Could you check a few things on this model? Use its own coordinates, in mm. A direction names the side the tool comes from. Round coordinates to 2 decimals unless told otherwise and drop trailing zeros. Loops run counter-clockwise (first coordinate to the right, second up) from the corner with the lowest first, then second, coordinate; pieces in that order, holes last. Notation, with made-up numbers: M 64,83 L 111,83 A28 cw 111,114 Z; hole C 2,55 d1. An arc over 180 degrees is marked long. Answer in a Markdown table with one row per item.
```python
from build123d import *

# Parameters (mm, degrees)
SKETCH_1_W          = 40
SKETCH_1_H          = 32
SKETCH_1_R          = 14
SKETCH_1_R_2        = 1.6
EXTRUDE_1_DEPTH     = 24
SKETCH_3_W          = 30.4
SKETCH_3_H          = 51.000805287
CUT_EXTRUDE_2_DEPTH = 22.4
SKETCH_4_W          = 6.12991639
SKETCH_4_H          = 19.114193836
CUT_EXTRUDE_3_DEPTH = 57.568542495
FILLET_1_R          = 1
SKETCH_6_W          = 15.6
SKETCH_6_H          = 32
EXTRUDE_3_DEPTH     = 10
SKETCH_8_R          = 1.6
CUT_EXTRUDE_4_DEPTH = 66.604877867
CUT_EXTRUDE_5_DEPTH = 66.604877867
CHAMFER_1_SIZE      = 1
SKETCH_10_W         = 3.521220791
SKETCH_10_H         = 7.290414878
CUT_EXTRUDE_6_DEPTH = 15
SKETCH_11_W         = 3.883261803
SKETCH_11_H         = 7.637577492
CUT_EXTRUDE_7_DEPTH = 11


with BuildPart() as part:
    # 草图1 → 凸台-拉伸1 (new body)
    with BuildSketch(Plane.XY):
        with Locations((-20, 16)):
            Rectangle(SKETCH_1_W, SKETCH_1_H)
        with Locations((-20, 16)):
            Circle(SKETCH_1_R, mode=Mode.SUBTRACT)
        with Locations((-2.64, 14.11)):
            Circle(SKETCH_1_R_2, mode=Mode.SUBTRACT)
        with Locations(Location((-37.36, 14.11, 0), (0, 0, 180))):
            Circle(SKETCH_1_R_2, mode=Mode.SUBTRACT)
    extrude(amount=EXTRUDE_1_DEPTH)

    # 草图3 → 切除-拉伸2 (cut)
    with BuildSketch(Plane(origin=(0, 0, 0), x_dir=(-1, 0, 0), z_dir=(0, 0, -1))):
        with Locations((20, 12.05288799)):
            Rectangle(SKETCH_3_W, SKETCH_3_H)
    extrude(amount=-CUT_EXTRUDE_2_DEPTH, mode=Mode.SUBTRACT)

    # 草图4 → 切除-拉伸3 (cut, through all)
    with BuildSketch(Plane(origin=(0, 0, 0), x_dir=(-1, 0, 0), z_dir=(0, 0, -1))):
        with Locations((0.535041805, 26.667096918)):
            Rectangle(SKETCH_4_W, SKETCH_4_H)
        with Locations((39.464958195, 26.667096918)):
            Rectangle(SKETCH_4_W, SKETCH_4_H)
        with Locations((39.464958195, 1.552903082)):
            Rectangle(SKETCH_4_W, SKETCH_4_H)
        with Locations((0.535041805, 1.552903082)):
            Rectangle(SKETCH_4_W, SKETCH_4_H)
    extrude(amount=-CUT_EXTRUDE_3_DEPTH, mode=Mode.SUBTRACT)

    # 圆角1
    fillet_1_edges = [part.edges().sort_by_distance(p)[0] for p in [
        (0, 11.11, 12),
        (0, 17.11, 12),
        (-40, 17.11, 12),
        (-40, 11.11, 12),
    ]]
    fillet(fillet_1_edges, radius=FILLET_1_R)

    # 草图6 → 凸台-拉伸3 (add)
    with BuildSketch(Plane.XY.offset(24)):
        with Locations((-44.2, 16)):
            Rectangle(SKETCH_6_W, SKETCH_6_H)
    extrude(amount=-EXTRUDE_3_DEPTH)

    # 草图8 → 切除-拉伸4 (cut, through all)
    with BuildSketch(Plane.XY.offset(24)):
        with Locations(Location((-37.36, 14.11, 0), (0, 0, 180))):
            Circle(SKETCH_8_R)
    extrude(amount=-CUT_EXTRUDE_4_DEPTH, mode=Mode.SUBTRACT)

    # 草图9 → 切除-拉伸5 (cut, through all)
    with BuildSketch(Plane(origin=(0, 32, 0), x_dir=(1, 0, 0), z_dir=(0, 1, 0))):
        Polygon((-51.102484963, -15.923925167), (-50.102484963, -14.923925167), (-42.006912692, -14.923925167), (-41.006912692, -15.923925167), (-41.006912692, -22.012190671), (-42.006912692, -23.012190671), (-50.102484963, -23.012190671), (-51.102484963, -22.012190671), align=None)
    extrude(amount=-CUT_EXTRUDE_5_DEPTH, mode=Mode.SUBTRACT)

    # 倒角1
    chamfer_1_edges = [part.edges().sort_by_distance(p)[0] for p in [
        (-52, 16, 24),
        (-52, 16, 14),
    ]]
    chamfer(chamfer_1_edges, length=CHAMFER_1_SIZE)

    # 草图10 → 切除-拉伸6 (cut)
    with BuildSketch(Plane(origin=(0, 32, 0), x_dir=(1, 0, 0), z_dir=(0, 1, 0))):
        with Locations((-38.274678112, -18.844062947)):
            Rectangle(SKETCH_10_W, SKETCH_10_H)
    extrude(amount=-CUT_EXTRUDE_6_DEPTH, mode=Mode.SUBTRACT)

    # 草图11 → 切除-拉伸7 (cut)
    with BuildSketch(Plane.XZ):
        with Locations((-38.341630902, 19.067238913)):
            Rectangle(SKETCH_11_W, SKETCH_11_H)
    extrude(amount=-CUT_EXTRUDE_7_DEPTH, mode=Mode.SUBTRACT)


solid = part.part
```
1) If we mould it in two halves opening along X, with no side actions, what happens to faces 1 (the face through (-38, 17, 19)), 2 (the face through (-46, 16, 23.012)), 3 (the face through (-37, 16, 0)), 4 (the face through (0, 14, 12))? For each: released by +X, released by -X, zero draft, split by the parting line, or undercut.
Computed:
| item | result |
|---|---|
| face 1 | undercut |
| face 2 | undercut |
| face 3 | zero draft |
| face 4 | released by +X |
2) Will these pins go through, and if not, where does the flat tip stop? P1, Ø4.5, axis at y = 14, z = 6.5, coming from the -X side; P2, Ø10, axis at x = -5.5, z = 7.5, coming from the -Y side; P3, Ø1.2, axis at x = -39, z = 20.5, coming from the -Y side; P4, Ø0.8, axis at x = -2.5, z = 14.5, coming from the -Y side.
Computed:
| item | result |
|---|---|
| P1 | stops at x = -40 |
| P2 | stops at y = 0 |
| P3 | stops at y = 11 |
| P4 | stops at y = 11.11 |
3) I want a section at C-C, the plane x = -2.64. Please give me the cut outline in (y, z).
Computed:
| item | result |
|---|---|
| outline | M 11.11,0 L 12.51,0 L 12.51,24 L 11.11,24 Z; M 15.71,0 L 17.11,0 L 17.11,24 L 15.71,24 Z |
4) I want a section at A-A, the plane z = 13. Please give me the cut outline in (x, y), plus the area to 3 significant figures.
Computed:
| item | result |
|---|---|
| outline | M -40,12.11 A1 ccw -39,11.11 L -36.4,11.11 L -36.4,0 L -35.2,0 L -35.2,32 L -36.4,32 L -36.4,17.11 L -39,17.11 A1 ccw -40,16.11 Z; M -4.8,0 L -3.6,0 L -3.6,11.11 L -1,11.11 A1 ccw 0,12.11 L 0,16.11 A1 ccw -1,17.11 L -3.6,17.11 L -3.6,32 L -4.8,32 Z; hole C -37.36,14.11 d3.2; hole C -2.64,14.11 d3.2 |
| area | 103 mm² |
5) I need wall thicknesses on line 1 (X direction, y = 1, z = 21.25); line 2 (X direction, y = 20, z = 17.25); line 3 (Z direction, x = -39, y = 28). Which ranges of each line are inside material? Lowest first, please.
Computed:
| item | result |
|---|---|
| line 1 | x = -52 to -51.1, -41.01 to -40.28, -36.4 to -35.2, -4.8 to -3.6 |
| line 2 | x = -52 to -51.1, -41.01 to -40.04, -36.51 to -35.2, -4.8 to -3.6 |
| line 3 | z = 14 to 15.2, 22.49 to 24 |
6) I want a section at D-D, the plane z = 20.25. Please give me the cut outline in (x, y), plus the area to 3 significant figures.
Computed:
| item | result |
|---|---|
| outline | M -52,0 L -51.1,0 L -51.1,32 L -52,32 Z; M -41.01,0 L -40.28,0 L -40.28,11 L -36.4,11 L -36.4,0 L -35.2,0 L -35.2,32 L -36.51,32 L -36.51,17 L -40.04,17 L -40.04,32 L -41.01,32 Z; M -4.8,0 L -3.6,0 L -3.6,11.11 L -1,11.11 A1 ccw 0,12.11 L 0,16.11 A1 ccw -1,17.11 L -3.6,17.11 L -3.6,32 L -4.8,32 Z; hole C -37.36,14.11 d3.2; hole C -2.64,14.11 d3.2 |
| area | 162 mm² |
7) I want a section at B-B, the plane y = 22. Please give me the cut outline in (x, z).
Computed:
| item | result |
|---|---|
| outline | M -52,15 L -51,14 L -36.4,14 L -36.4,0 L -35.2,0 L -35.2,22.4 L -32.65,22.4 L -32.65,24 L -51,24 L -52,23 Z; M -7.35,22.4 L -4.8,22.4 L -4.8,0 L -3.6,0 L -3.6,24 L -7.35,24 Z; hole M -51.1,15.92 L -50.1,14.92 L -42.01,14.92 L -41.01,15.92 L -41.01,22.01 L -42.01,23.01 L -50.1,23.01 L -51.1,22.01 Z; hole M -40.04,15.2 L -36.51,15.2 L -36.51,22.49 L -40.04,22.49 Z |
8) Which directions (+Z, -Z, +X, -X, +Y, -Y) give clear straight access to the entire face, cutting with the end or side of a thin tool? Please do faces 5 (the face through (-41.5, 16.224, 22.505)), 6 (the face through (-4.8, 16, 11)), 7 (the face through (-3.6, 24, 12)), 8 (the face through (-38, 11, 19)), 9 (the face through (-36.4, 24, 7)).
Computed:
| item | result |
|---|---|
| face 5 | +Y, -Y |
| face 6 | -Z, +Y, -Y |
| face 7 | +Z, -Z, +X, +Y |
| face 8 | -Y |
| face 9 | -Z, -X, +Y |
